Input: dimensioned drawing with shaded views. Units: mm. Origin: part minimum x, y, z. Round coordinates to 2 decimals unless told otherwise and drop trailing zeros. Order: outer loops, then holes, each group sorted by start corner. A loop starts at its lowest first (then second) coordinate and runs counter-clockwise, first axis right, second up. Notation, with made-up numbers: M 46.25,8.25 L 70.25,8.25 A30 cw 70.25,30.25 Z; hole C -26.75,45 d11. An arc over 180 degrees is marked long. Answer as CSV lines item,"result". Start each with the question number.
Item 1: First-contact query: P1, Ø5, axis at x = 27.5, z = 10, coming from the -Y side. Flat tip, straight axial feed; report the tip coordinate or a pass-through.
Item 2: Section query C-C on y = 1.8. Return the cut outline in (x, z).
Item 3: Line query: line 1 (X direction, y = 2.45, z = 7.25); line 2 (Z direction, x = 42.5, y = 1.25); line 3 (Z direction, x = 50.5, y = 0.6). Output: solid intervals per line, ascending. Write a range as [from, to].
Item 4: Section query A-A on x = 27.5. Return the cut outline in (y, z), plus the area to 3 significant figures.
Item 5: Section query B-B on z = 10. Return the cut outline in (x, y).
Item 6: Section query D-D on x = 60. Return the cut outline in (y, z), plus the area to 3 significant figures.
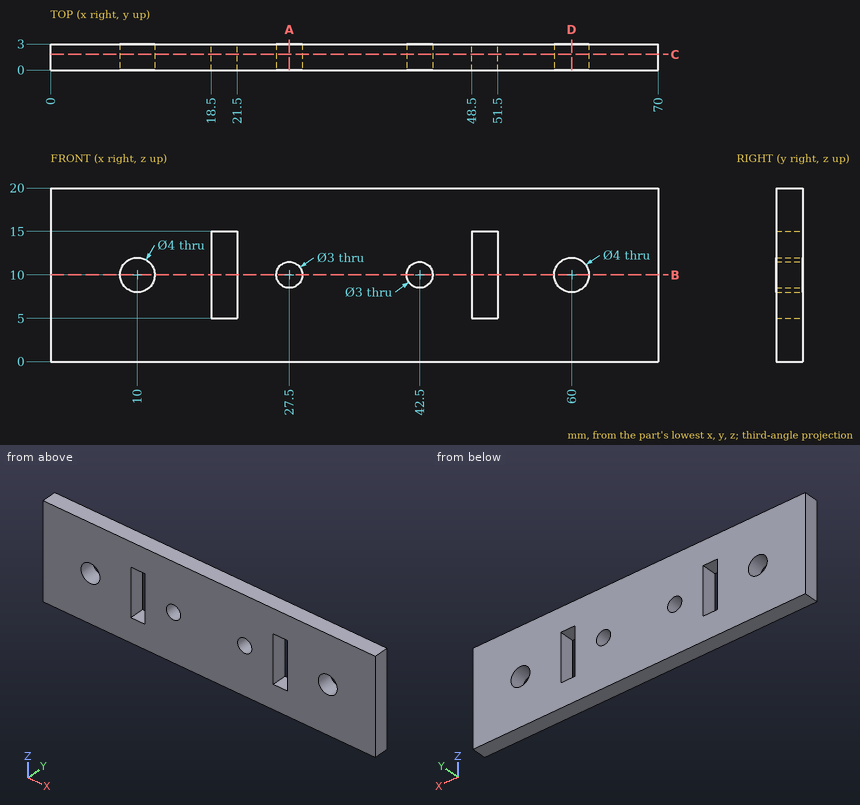
Results:
1,P1,"y = 0"
2,outline,"M 0,0 L 70,0 L 70,20 L 0,20 Z; hole C 10,10 d4; hole M 18.5,5 L 21.5,5 L 21.5,15 L 18.5,15 Z; hole C 27.5,10 d3; hole C 42.5,10 d3; hole M 48.5,5 L 51.5,5 L 51.5,15 L 48.5,15 Z; hole C 60,10 d4"
3,line 1,"[0, 18.5], [21.5, 48.5], [51.5, 70]"
3,line 2,"[0, 8.5], [11.5, 20]"
3,line 3,"[0, 5], [15, 20]"
4,outline,"M 0,0 L 3,0 L 3,8.5 L 0,8.5 Z; M 0,11.5 L 3,11.5 L 3,20 L 0,20 Z"
4,area,"51.0 mm^2"
5,outline,"M 0,0 L 8,0 L 8,3 L 0,3 Z; M 12,0 L 18.5,0 L 18.5,3 L 12,3 Z; M 21.5,0 L 26,0 L 26,3 L 21.5,3 Z; M 29,0 L 41,0 L 41,3 L 29,3 Z; M 44,0 L 48.5,0 L 48.5,3 L 44,3 Z; M 51.5,0 L 58,0 L 58,3 L 51.5,3 Z; M 62,0 L 70,0 L 70,3 L 62,3 Z"
6,outline,"M 0,0 L 3,0 L 3,8 L 0,8 Z; M 0,12 L 3,12 L 3,20 L 0,20 Z"
6,area,"48.0 mm^2"
